Can you work these out from the model? Positions are in its coordinate system, mm. Face numbers are marked on the shaded views. A direction names the side the tool comes from. Give positions to 0.01 mm unless a question says otherwise; leave off trailing zeros. Write each loop counter-clockwise with the first axis right and the second up, starting at its lowest first coordinate (ties: lowest second). Pieces come first, ordered by that corner, then holes.
1. Suppose I cut it at B-B (y = 64). Please give me the cut outline in (x, z).
2. On a 3-axis mill with a long thin cutter (end or side, diameter ignored), from which of +Z, -Z, +X, -X, +Y, -Y can I reach the whole of each face in a straight line? I mean the marked faces 3, 4 and 5. Say none if no direction works.
3. Suppose I cut it at C-C (z = -71). Please give me the cut outline in (x, y).
4. Thinking about a two-plate mould opening in Z: for the marked faces 1 and 2, which applies, pulls with the +Z half, pulls with the -Z half, needs draft (parallel to the pull), parting line crosses it, or undercut?
5. I'm going to push flat-ended pins straight in: pin 1 (8 mm diameter, centred on x = 7.5, z = -24, fed in from -Y); pin 2 (4 mm diameter, centred on x = 7, z = 34.5, fed in from +Y); pin 3 (5 mm diameter, centred on x = -20.5, y = -34.5, fed in from +Z); pin 4 (17 mm diameter, centred on x = 1, z = -44.5, fed in from +Y). Where does each tip first touch, or does it pass through?
6. Suppose I cut it at D-D (y = -28.5). Please give me the cut outline in (x, z), and give its area (3 significant figures).
7. If I drill on probe 1 along Z at (x, y) = (36, 0); probe 2 along Z at (x, y) = (-26, 0); probe 3 along Z at (x, y) = (11, 0), over which ranges is the centre line in solid material (lowest first)?
8. Suppose I cut it at A-A (x = 31). Give the number of separate pieces and of enclosed holes in the cut face, and give its area (3 significant figures).
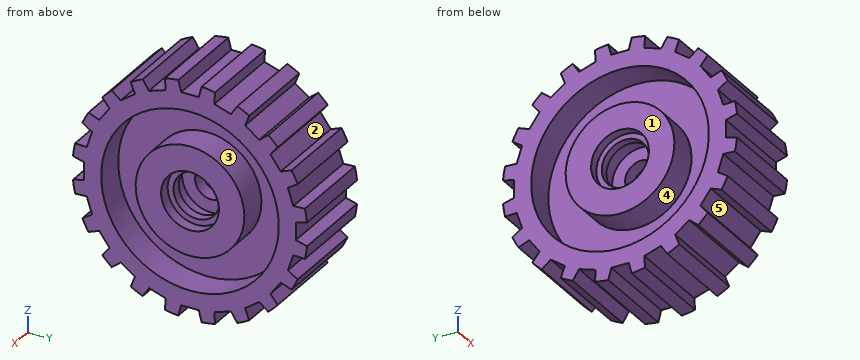
```python
from build123d import *

# Parameters (mm, degrees)
F3_DEPTH        = 88.646
F3_COPIES_COUNT = 20


# Not quite as in the source:
# - a feature of the source that left no trace in its solid (it failed there, or was rolled back) is left out
# - a pattern or mirror of a feature is missing from the dataset's text; its kind, count and spacing are read off the source's solid


with BuildPart() as f1:
    # F0 (on Front) → F1 (revolve)
    with BuildSketch(Plane.XZ):
        Polygon((38.1, 36.1084090909), (38.1, 61.5084090909), (-38.1, 61.5084090909), (-38.1, 36.1084090909), (-11.9062505468, 36.1084090909), (-11.9062505468, 5.6284090909), (-38.1, 5.6284090909), (-38.1, -16.8852278195), (-30.0903403623, -16.8852278195), (-30.0903403623, -21.6477272727), (-22.9465920027, -21.6477272727), (-22.9465920027, -16.8852278195), (-6.0613630896, -16.8852278195), (-6.0613630896, -28.3585221805), (6.0613652768, -28.3585221805), (6.0613652768, -16.8852278195), (20.1323869104, -16.8852278195), (20.1323869104, -22.0806807246), (28.1420443609, -22.0806807246), (28.1420443609, -16.8852278195), (38.1, -16.8852278195), (38.1, 5.6284090909), (12.1227261791, 5.6284090909), (12.1227261791, 36.1084090909), align=None)
    revolve(axis=Axis((0.8659090909, 0, -42.4295432673), (1, 0, 0)))

    # F2 (on face) → F3 (cut, symmetric)
    with BuildSketch(Plane.YZ.offset(28.1420443609)):
        Polygon((0, 65.8745542169), (-11.6578890011, 65.8745542169), (-7.7292122878, 51.0664619505), (0, 51.0664619505), (7.7292122878, 51.0664619505), (11.6578890011, 65.8745542169), align=None)
    f3 = extrude(amount=F3_DEPTH, both=True, mode=Mode.SUBTRACT)

    # F3_copies: F3 ×20 about axis
    f3_copies_axis = Axis((0, 0, -42.429543), (1, 0, 0))
    for i in range(1, F3_COPIES_COUNT):
        add(f3.rotate(f3_copies_axis, i * 360 / F3_COPIES_COUNT), mode=Mode.SUBTRACT)


solid = f1.part
```
Checks:
1. outline: (-38.1, -115.8) - (38.1, -115.8) - (38.1, -87.95) - (12.12, -87.95) - (12.12, 3.09) - (38.1, 3.09) - (38.1, 30.94) - (-38.1, 30.94) - (-38.1, 3.09) - (-11.91, 3.09) - (-11.91, -87.95) - (-38.1, -87.95) - close
2. face 3: +X
2. face 4: -X
2. face 5: +X, -X
3. outline: (-38.1, -89.02) - (38.1, -89.02) - (38.1, -73.16) - (12.12, -73.16) - (12.12, -38.64) - (38.1, -38.64) - (38.1, 38.64) - (12.12, 38.64) - (12.12, 73.16) - (38.1, 73.16) - (38.1, 89.02) - (-38.1, 89.02) - (-38.1, 73.16) - (-11.91, 73.16) - (-11.91, 38.64) - (-38.1, 38.64) - (-38.1, -38.64) - (-11.91, -38.64) - (-11.91, -73.16) - (-38.1, -73.16) - close
4. face 1: needs draft
4. face 2: undercut
5. pin 1: stops at y = -102.93
5. pin 2: stops at y = 72.03
5. pin 3: stops at z = 45.48
5. pin 4: stops at y = 103.42
6. outline: (-38.1, -131.48) - (38.1, -131.48) - (38.1, -115.61) - (12.12, -115.61) - (12.12, -81.12) - (38.1, -81.12) - (38.1, -3.73) - (12.12, -3.73) - (12.12, 30.75) - (38.1, 30.75) - (38.1, 46.62) - (-38.1, 46.62) - (-38.1, 30.75) - (-11.91, 30.75) - (-11.91, -3.73) - (-38.1, -3.73) - (-38.1, -81.12) - (-11.91, -81.12) - (-11.91, -115.61) - (-38.1, -115.61) - close
6. area: 9,970 mm2
7. probe 1: z = -135.93 to -120.97, -90.49 to -67.97, -16.89 to 5.63, 36.11 to 51.07
7. probe 2: z = -135.93 to -120.97, -90.49 to -63.21, -21.65 to 5.63, 36.11 to 51.07
7. probe 3: z = -135.93 to -67.97, -16.89 to 51.07
8. separate pieces: 2
8. enclosed holes: 2
8. area: 16,000 mm2
